from build123d import *

# Parameters (mm, degrees)
F0_W     = 31.75
F0_H     = 25.4
F1_DEPTH = 11.1125
F2_W     = 11.1125
F2_H     = 31.75
F3_DEPTH = 3.175
F4_W     = 11.1125
F4_H     = 25.4
F5_DEPTH = 6.35


with BuildPart() as f1:
    # F0 (on Front) → F1 (new body)
    with BuildSketch(Plane.XZ):
        with Locations((-13.603202, -30.109987)):
            Rectangle(F0_W, F0_H)
    extrude(amount=F1_DEPTH)

    # F2 (on face) → F3 (join)
    with BuildSketch(Plane.YZ.offset(2.271798)):
        with Locations((-5.55625, -30.109987)):
            Rectangle(F2_W, F2_H)
    extrude(amount=F3_DEPTH)

    # F4 (on face) → F5 (join)
    with BuildSketch(Plane.YZ.offset(5.446798)):
        with Locations((-5.55625, -30.109987)):
            Rectangle(F4_W, F4_H)
    extrude(amount=F5_DEPTH)


solid = f1.part
The listing builds one solid part. Answer for the finished solid, in the listing's coordinates (mm). A direction names the side the tool comes from. Round coordinates to 2 decimals unless told otherwise and drop trailing zeros. Order: outer loops, then holes, each group sorted by start corner. A loop starts at its lowest first (then second) coordinate and runs counter-clockwise, first axis right, second up. Notation, with made-up numbers: (-33, 67) -> (3, 67) arc R24 cw to (3, 99) -> close; hole circle Ø1 at (41, 58.5). An arc over 180 degrees is marked (long way). One line per item, written item: value.
Item 1: For faces 1 (the flat face through (5.447, -6, -44)), 2 (the flat face through (5.447, -6, -16)), 3 (the flat face through (-14, -5, -17.41)), determine the directions among +Z, -Z, +X, -X, +Y, -Y from which every point of the face is accessible in a straight line to the end or side of a thin tool.
Taken from the geometry:
face 1: -Z, +X, +Y, -Y
face 2: +Z, +X, +Y, -Y
face 3: +Z, -X, +Y, -Y
Item 2: Find section A-A, the plane y = -5. Give the vertices of the cut face in (x, z).
Taken from the geometry:
outline: (-29.48, -42.81) -> (2.27, -42.81) -> (2.27, -45.98) -> (5.45, -45.98) -> (5.45, -42.81) -> (11.8, -42.81) -> (11.8, -17.41) -> (5.45, -17.41) -> (5.45, -14.23) -> (2.27, -14.23) -> (2.27, -17.41) -> (-29.48, -17.41) -> close
Item 3: Given P1, Ø4, axis at x = -9, y = -4, coming from the -Z side; P2, Ø4, axis at x = -19, y = -6, coming from the +Z side; P3, Ø1, axis at y = -4.5, z = -15.5, coming from the +X side, each flat-ended and moving along its own axis, determine where each tip first touches the part or whether it passes through.
Taken from the geometry:
P1: stops at z = -42.81
P2: stops at z = -17.41
P3: stops at x = 5.45
Item 4: Find section B-B, the plane x = -13.5. Give the vertices of the cut face in (y, z).
Taken from the geometry:
outline: (-11.11, -42.81) -> (0, -42.81) -> (0, -17.41) -> (-11.11, -17.41) -> close
Item 5: Straight lines are drawn through the part: L1, parallel to X at y = -9.25, z = -43.5; L2, parallel to Z at x = -26, y = -2.75. For each, find the intervals that lie inside material, in ascending order.
Taken from the geometry:
L1: x = 2.27 to 5.45
L2: z = -42.81 to -17.41
